Could you check a few things on this model? Use its own coordinates, in mm. Face numbers are marked on the shaded views. A direction names the side the tool comes from. Round coordinates to 2 decimals unless told otherwise and drop trailing zeros. Order: outer loops, then holes, each group sorted by start corner. A loop starts at its lowest first (then second) coordinate and runs counter-clockwise, first axis right, second up. Notation, with made-up numbers: (81.25, 28) -> (136.25, 28) arc R12 ccw to (136.25, 49) -> close; hole circle Ø4 at (62, -13.5). An arc over 180 degrees is marked (long way). One line per question, with ' | ' between items.
```python
from build123d import *

# Parameters (mm, degrees)
F0_R      = 19.05
F2_DEPTH  = 15.875
F1_R      = 9.525
F3_DEPTH  = 15.24
F4_R      = 1.5875
F5_DEPTH  = 1.5875
F6_R      = 3.175
F7_DEPTH  = 7.9375
F9_R      = 1.5875
F10_DEPTH = 25.4


with BuildPart() as f2:
    # F0 (on Front) → F2 (new body)
    with BuildSketch(Plane.XZ):
        Circle(F0_R)
    extrude(amount=-F2_DEPTH)

    # F1 (on face) → F3 (cut)
    with BuildSketch(Plane.XZ):
        Circle(F1_R)
    extrude(amount=-F3_DEPTH, mode=Mode.SUBTRACT)

    # F4 (on face) → F5 (join)
    with BuildSketch(Plane.XZ.offset(-15.24)):
        Circle(F4_R)
    extrude(amount=F5_DEPTH)

    # F6 (on face) → F7 (join)
    with BuildSketch(Plane(origin=(0, 15.875, 0), x_dir=(-1, 0, 0), z_dir=(0, 1, 0))):
        Circle(F6_R)
    extrude(amount=F7_DEPTH)

    # F9 (on face) → F10 (cut)
    with BuildSketch(Plane(origin=(0, 15.875, 0), x_dir=(-1, 0, 0), z_dir=(0, 1, 0))):
        with Locations((6.35, 0)):
            Circle(F9_R)
        with Locations((4.490128, 4.490128)):
            Circle(F9_R)
        with Locations((0, 6.35)):
            Circle(F9_R)
        with Locations((-4.490128, 4.490128)):
            Circle(F9_R)
        with Locations((-6.35, 0)):
            Circle(F9_R)
        with Locations((-4.490128, -4.490128)):
            Circle(F9_R)
        with Locations((0, -6.35)):
            Circle(F9_R)
        with Locations((4.490128, -4.490128)):
            Circle(F9_R)
    extrude(amount=-F10_DEPTH, mode=Mode.SUBTRACT)


solid = f2.part
```
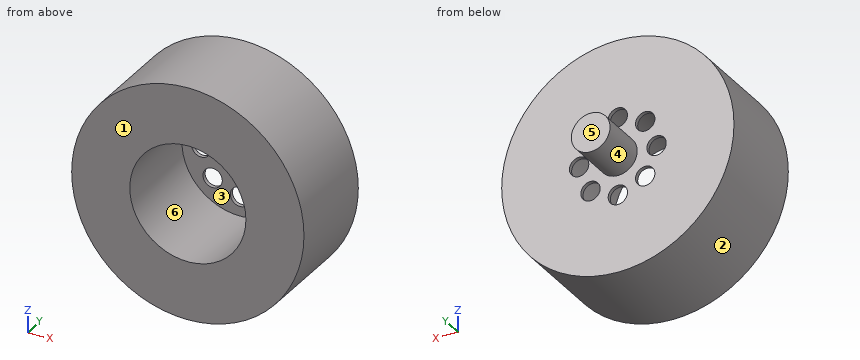
1. I want a section at C-C on x = 5.5. List the corners of the cut face in (y, z) for me (3 decimals), and give its area (3 significant figures).
From the geometry:
outline: (0, -18.239) -> (15.875, -18.239) -> (15.875, -5.715) -> (15.24, -5.715) -> (15.24, -7.777) -> (0, -7.777) -> close; (0, 7.777) -> (15.24, 7.777) -> (15.24, 5.715) -> (15.875, 5.715) -> (15.875, 18.239) -> (0, 18.239) -> close; (15.24, -3.265) -> (15.875, -3.265) -> (15.875, -1.341) -> (15.24, -1.341) -> close; (15.24, 1.341) -> (15.875, 1.341) -> (15.875, 3.265) -> (15.24, 3.265) -> close | area: 337 mm²
2. On a 3-axis mill with a long thin cutter (end or side, diameter ignored), from which of +Z, -Z, +X, -X, +Y, -Y can I reach the whole of each face in a straight line? I mean the marked faces 4, 5 and 6. Say none if no direction works.
From the geometry:
face 4: +Y | face 5: +Z, -Z, +X, -X, +Y | face 6: -Y
3. I want a section at D-D on y = 11.75. List the corners of the cut face in (x, z) for me (3 decimals), and give its area (3 significant figures).
From the geometry:
outline: circle Ø38.1 at (0, 0); hole circle Ø19.05 at (0, 0) | area: 855 mm²
4. I need wall thicknesses on probe 1 along Z at (x, y) = (0, 15.4); probe 2 along Y at (x, z) = (-2.5, 14) (3 decimals); probe 3 along Z at (x, y) = (0, 4.5) (3 decimals). Which ranges of each line are inside material? Lowest first, please.
From the geometry:
probe 1: z = -19.05 to -7.94, -4.76 to 4.76, 7.94 to 19.05 | probe 2: y = 0 to 15.875 | probe 3: z = -19.05 to -9.525, 9.525 to 19.05
5. I want a section at A-A on x = 0. Count the separate pieces of the cut face and the enclosed holes in it, and give its area (3 significant figures).
From the geometry:
separate pieces: 3 | enclosed holes: 0 | area: 366 mm²
6. I'm going to push flat-ended pins straight in: pin 1 (5 mm diameter, centred on x = 0, z = 6.35, fed in from +Y) (3 decimals); pin 2 (5 mm diameter, centred on x = 3, z = -6, fed in from -Y); pin 3 (2 mm diameter, centred on x = -2.5, y = 13, fed in from +Z); pin 4 (1.9 mm diameter, centred on x = 0, z = -6.35, fed in from +Y). Where does each tip first touch, or does it pass through?
From the geometry:
pin 1: stops at y = 15.875 | pin 2: stops at y = 15.24 | pin 3: stops at z = 18.99 | pin 4: passes through
7. If we mould it in two halves opening along Z, with no side actions, what happens to the marked faces 1, 2 and 3? For each: pulls with the +Z half, pulls with the -Z half, needs draft (parallel to the pull), parting line crosses it, or undercut.
From the geometry:
face 1: needs draft | face 2: parting line crosses it | face 3: undercut
